Autodesk Inventor part; units mm, degrees
ref_plane "Plan YZ" through (0, 0, 0) normal (1, 0, 0) x (0, 1, 0)
ref_plane "Plan XZ" through (0, 0, 0) normal (0, 1, 0) x (-1, 0, 0)
ref_plane "Plan XY" through (0, 0, 0) normal (0, 0, 1) x (1, 0, 0)
sketch "Esquisse1" plane through (0, 0, 0) normal (0, 0, 1) x (1, 0, 0)
  circle A0 centre (0, 0) radius 4
  dimension "d0" = 8
extrude "Extrusion1" add sketch "Esquisse1" along normal blind 75
sketch "Esquisse6" plane through (0, 0, 75) normal (0, 0, 1) x (1, 0, 0)
  point P0 (0, 0)
  point P1 (0, 0)
hole "Perçage1" at (0, 0, 75) direction (0, 0, -1) diameter 2.459 depth 8.5 tip angle 118
sketch "Esquisse7" plane through (0, 0, 0) normal (0, 0, -1) x (-1, 0, 0)
  circle A0 centre (0, 0) radius 1.2295
hole "Perçage2" at (0, 0, 0) direction (0, 0, 1) diameter 2.459 depth 8.5 tip angle 118
chamfer "Chanfrein1" distance 0.5 angle 45 2 edges at (-4, 0, 0) (-4, 0, 75)
properties part number "P1704_001" material ".EN AW-6082/AlMgSi1"
Check sheet for the modelled part. Datum: model origin and axes. Units: mm. A direction names the side the tool comes from. Round coordinates to 2 decimals unless told otherwise and drop trailing zeros. Loops run counter-clockwise (first coordinate to the right, second up) from the corner with the lowest first, then second, coordinate; pieces in that order, holes last. Notation, with made-up numbers: (15, 65) - (50, 65) arc R21 cw to (50, 80) - close; hole circle Ø1 at (-19.75, 72.25). An arc over 180 degrees is marked (long way). Answer as a JSON object with one key per item and string values. Group by question number.
Q1. Mould release check, pull along X, two halves, no side actions. Record for faces 1 (the face through (0.748, -0.976, 4.31)), 2 (the face through (0, -2, 0)), 3 (the face through (-0.867, 3.905, 36.982)): released by +X, released by -X, zero draft, split by the parting line, or undercut.
Q2. Gauge pin test, flat ends, axial feed: P1, Ø1, axis at y = 1, z = 14.5, coming from the -X side; P2, Ø1, axis at y = -3, z = 40, coming from the +X side. Record the tip position at first contact, or that the pin passes through.
Q3. Scan lines: line 1 along Y through (x, z) = (0, 70.5); line 2 along X through (y, z) = (0.25, 36); line 3 along Y through (x, z) = (1.5, 66.5). Record each from-to range of solid material in increasing order. Write a range as [from, to].
Q4. Set-up check for faces 4 (the face through (0, -2, 75)), 5 (the face through (0.748, 0.976, 70.69)): record each of +Z, -Z, +X, -X, +Y, -Y from which the full face is reachable in a straight line by a thin tool's end or side.
Q5. Sectioned sample at A-A, the plane z = 53.5. Enter the section's corners in (x, y).
Solution:
{
 "1": {"face 1": "undercut", "face 2": "zero draft", "face 3": "split by the parting line"},
 "2": {"P1": "stops at x = -3.97", "P2": "stops at x = 3.12"},
 "3": {"line 1": "y = [-4, -1.23], [1.23, 4]", "line 2": "x = [-3.99, 3.99]", "line 3": "y = [-3.71, 3.71]"},
 "4": {"face 4": "+Z, +X, -X, +Y, -Y", "face 5": "+Z"},
 "5": {"outline": "circle Ø8 at (0, 0)"}
}
